The model under review builds one solid part; all positions refer to its coordinate system, in mm. Face numbers are marked on the shaded views. A direction names the side the tool comes from. Round coordinates to 2 decimals unless told otherwise and drop trailing zeros. Order: outer loops, then holes, each group sorted by start corner. A loop starts at its lowest first (then second) coordinate and runs counter-clockwise, first axis right, second up.
1) Mouldability with a two-part tool opening along X and no side actions: class the marked faces 3, 4 and 5 as pulls with the +X half, pulls with the -X half, needs draft (parallel to the pull), parting line crosses it, or undercut.
2) Clearance check with flat-ended pins moving along their axes: P1, Ø4, axis at x = -23.5, z = 21.5, coming from the +Y side; P2, Ø5, axis at x = 10.5, y = -6, coming from the +Z side. State where each tip first meets the part, or that it passes through.
3) Consider section D-D (x = -2). Give the boundary of the cut face in (y, z).
4) Consider section C-C (y = -10). Give the boundary of the cut face in (x, z).
5) Consider section B-B (x = -20). Give the boundary of the cut face in (y, z), then the cut area to 3 significant figures.
6) Machinability: for the marked faces 1 and 2, which of the approach directions +Z, -Z, +X, -X, +Y, -Y give a long, thin tool a straight path to every point of the face, cutting with its end or side? Answer none if there is none.
7) To check wall thickness, follow L1, parallel to Z at x = -2, y = -11.5; L2, parallel to X at y = 3.5, z = 31; L3, parallel to X at y = -5.5, z = 31. State the ranges of each line that lie inside material, in increasing order.
8) Consider section A-A (y = 0). Give the boundary of the cut face in (x, z), then the cut area to 3 significant figures.
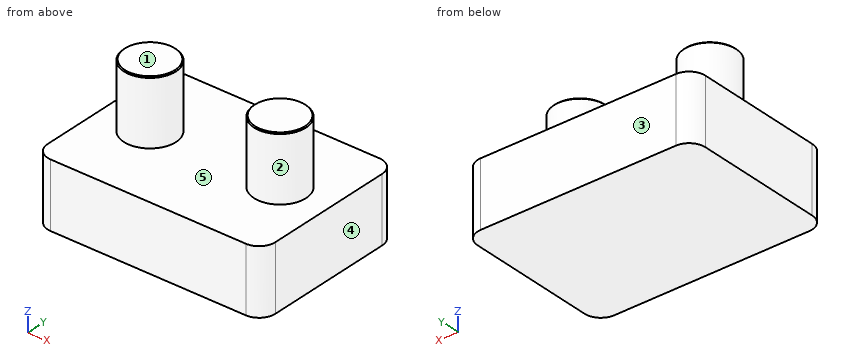
from build123d import *

# Parameters (mm, degrees)
SKETCH_1_W      = 70
SKETCH_1_H      = 50
EXTRUDE_1_DEPTH = 20
SKETCH_2_R      = 8
EXTRUDE_2_DEPTH = 20
CHAMFER_1_SIZE  = 0.3
FILLET_1_R      = 5


with BuildPart() as part:
    # Sketch 1 → Extrude 1 (new body)
    with BuildSketch(Plane.XY):
        Rectangle(SKETCH_1_W, SKETCH_1_H)
    extrude(amount=EXTRUDE_1_DEPTH)

    # Sketch 2 → Extrude 2 (add)
    with BuildSketch(Plane.XY.offset(20)):
        with Locations(Location((-20, 0, 0), (0, 0, 180))):
            Circle(SKETCH_2_R)
        with Locations(Location((20, 0, 0), (0, 0, 180))):
            Circle(SKETCH_2_R)
    extrude(amount=EXTRUDE_2_DEPTH)

    # Chamfer 1
    chamfer_1_edges = [part.edges().sort_by_distance(p)[0] for p in [
        (-12, 0, 40),
        (28, 0, 40),
    ]]
    chamfer(chamfer_1_edges, length=CHAMFER_1_SIZE)

    # Fillet 1
    fillet_1_edges = [part.edges().sort_by_distance(p)[0] for p in [
        (-35, 25, 10),
        (35, 25, 10),
        (35, -25, 10),
        (-35, -25, 10),
    ]]
    fillet(fillet_1_edges, radius=FILLET_1_R)


solid = part.part
Answer below:
1. face 3: needs draft
1. face 4: pulls with the +X half
1. face 5: undercut
2. P1: stops at y = 25
2. P2: stops at z = 20
3. outline: (-25, 0) - (25, 0) - (25, 20) - (-25, 20) - close
4. outline: (-35, 0) - (35, 0) - (35, 20) - (-35, 20) - close
5. outline: (-25, 0) - (25, 0) - (25, 20) - (8, 20) - (8, 39.7) - (7.7, 40) - (-7.7, 40) - (-8, 39.7) - (-8, 20) - (-25, 20) - close
5. area: 1,320 mm2
6. face 1: +Z, +X, -X, +Y, -Y
6. face 2: +Z
7. L1: z = 0 to 20
7. L2: x = -27.19 to -12.81, 12.81 to 27.19
7. L3: x = -25.81 to -14.19, 14.19 to 25.81
8. outline: (-35, 0) - (35, 0) - (35, 20) - (28, 20) - (28, 39.7) - (27.7, 40) - (12.3, 40) - (12, 39.7) - (12, 20) - (-12, 20) - (-12, 39.7) - (-12.3, 40) - (-27.7, 40) - (-28, 39.7) - (-28, 20) - (-35, 20) - close
8. area: 2,040 mm2
